Study the drawing (mm; zero at the part's minimum x, y, z) and answer. Give positions to 0.01 mm unless a question says otherwise; leave off trailing zeros. Order: outer loops, then holes, each group sorted by start corner. A loop starts at its lowest first (then second) coordinate and runs counter-clockwise, first axis right, second up. Notation, with made-up numbers: (62.5, -3) - (87.5, -3) arc R17 cw to (87.5, 22) - close; hole circle Ø11 at (77.25, 7.25). An arc over 180 degrees is marked (long way). Put each result on its own line as item: value.
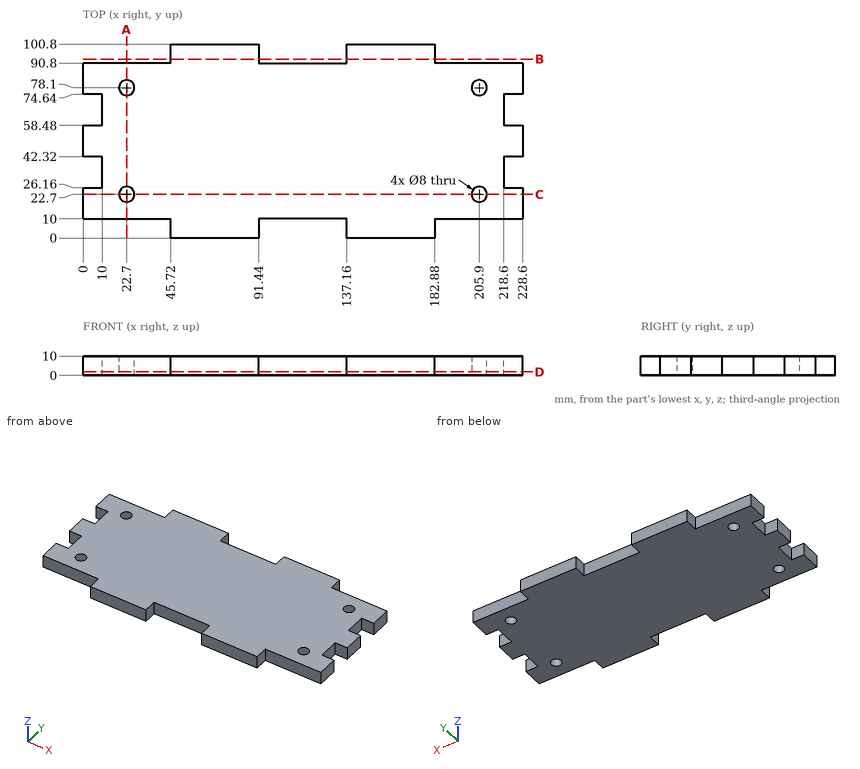
(1) Straight lines are drawn through the part: line 1 (Y direction, x = 22.7, z = 3.5); line 2 (X direction, y = 78, z = 7); line 3 (X direction, y = 91.5, z = 0.5). For each, find the intervals that lie inside material, in ascending order.
Geometry check:
line 1: y = 10 to 18.7, 26.7 to 74.1, 82.1 to 90.8
line 2: x = 0 to 18.7, 26.7 to 201.9, 209.9 to 228.6
line 3: x = 45.72 to 91.44, 137.16 to 182.88
(2) Section D-D, the plane z = 1.75 is taken. Count the separate pieces of the cut face and the enclosed holes in it, then the cut area to 3 significant figures.
Geometry check:
separate pieces: 1
enclosed holes: 4
area: 19,500 mm²
(3) Section B-B, the plane y = 93 is taken. Write down the section's boundary in (x, z).
Geometry check:
outline: (45.72, 0) - (91.44, 0) - (91.44, 10) - (45.72, 10) - close; (137.16, 0) - (182.88, 0) - (182.88, 10) - (137.16, 10) - close
(4) Given pin 1 (3 mm diameter, centred on y = 73, z = 7.5, fed in from -X); pin 2 (3 mm diameter, centred on x = 114.5, z = 7, fed in from -Y); pin 3 (5 mm diameter, centred on x = 222, z = 4.5, fed in from +Y), each flat-ended and moving along its own axis, determine where each tip first touches the part or whether it passes through.
Geometry check:
pin 1: stops at x = 10
pin 2: stops at y = 10
pin 3: stops at y = 90.8
(5) Section A-A, the plane x = 22.7 is taken. Write down the section's boundary in (y, z).
Geometry check:
outline: (10, 0) - (18.7, 0) - (18.7, 10) - (10, 10) - close; (26.7, 0) - (74.1, 0) - (74.1, 10) - (26.7, 10) - close; (82.1, 0) - (90.8, 0) - (90.8, 10) - (82.1, 10) - close
(6) Section C-C, the plane y = 22.7 is taken. Write down the section's boundary in (x, z), then the cut area to 3 significant figures.
Geometry check:
outline: (0, 0) - (18.7, 0) - (18.7, 10) - (0, 10) - close; (26.7, 0) - (201.9, 0) - (201.9, 10) - (26.7, 10) - close; (209.9, 0) - (228.6, 0) - (228.6, 10) - (209.9, 10) - close
area: 2,130 mm²
